CAD build for the part. Positions are in the model's coordinates, mm. A direction names the side the tool comes from. Round coordinates to 2 decimals unless told otherwise and drop trailing zeros. Order: outer loops, then holes, each group sorted by start corner. A loop starts at its lowest first (then second) coordinate and runs counter-clockwise, first axis right, second up. Notation, with made-up numbers: (88, 22) -> (135, 22) arc R14 ccw to (135, 48) -> close; hole circle Ø1 at (4, 28.5). An arc over 180 degrees is marked (long way). Return JSON: item names as keys, results as strings. Group by question number.
Q1. Flat gauge pins, fed straight in: pin 1 (1 mm diameter, centred on x = 54, z = 1.5, fed in from +Y); pin 2 (1 mm diameter, centred on y = 3.5, z = 1, fed in from -X); pin 3 (1.8 mm diameter, centred on y = 4.5, z = 2.5, fed in from +X); pin 4 (3 mm diameter, centred on x = 9.5, z = 2.5, fed in from +Y). Where does each tip first touch, or does it go through?
Q2. Cut at D-D (x = 5). Write the cut outline in (y, z), then the cut area to 3 significant figures.
Q3. Cut at C-C (x = 70). Write the cut outline in (y, z), then the cut area to 3 significant figures.
Q4. Cut at B-B (y = 33). Write the cut outline in (x, z).
Q5. Cut at A-A (z = 2). Write the cut outline in (x, y).
Q6. Probe line 1 along X through (y, z) = (4.5, 0.75); line 2 along Y through (x, z) = (70, -1); line 3 along Y through (x, z) = (5, -0.85). List the from-to ranges inside material, lowest first.
Q7. Which spindle directions (+Z, -Z, +X, -X, +Y, -Y) get a long thin tool onto all of the face, cutting with end or side? Do faces 1 (the flat face through (44.5, 12, 2)), 2 (the cylindrical face through (56.669, 19.474, 6.458)), 3 (the flat face through (55, 23, 2)). Say none if no direction does.
Q8. Mould opens along Y. For faces 4 (the flat face through (53.6, 18.7, 3.5)), 5 (the cylindrical face through (56.617, 5.67, 6.458)), 6 (the flat face through (47, 13, 9.5)), 7 (the flat face through (47, 15.5, 2)) say: +Y half, -Y half, draft (parallel to the pull), parting line (faces both ways), or undercut.
Autodesk Inventor part; units mm, degrees
ref_plane "YZ Plane" through (0, 0, 0) normal (1, 0, 0) x (0, 1, 0)
ref_plane "XZ Plane" through (0, 0, 0) normal (0, 1, 0) x (-1, 0, 0)
ref_plane "XY Plane" through (0, 0, 0) normal (0, 0, 1) x (1, 0, 0)
sketch "Skizze1" plane through (0, 0, 0) normal (0, 0, 1) x (1, 0, 0)
  line L0 (0, 0) -> (90, 0)
  line L1 (90, 0) -> (90, 37)
  line L2 (90, 37) -> (0, 37)
  line L3 (0, 37) -> (0, 0)
  dimension "d0" = 90
  dimension "d1" = 37
extrude "Extrusion1" add sketch "Skizze1" against normal blind 1.6
sketch "Skizze2" plane through (0, 0, 0) normal (0, 0, 1) x (1, 0, 0)
  circle A0 centre (5, 33) radius 1.75
  circle A1 centre (37.5, 5) radius 1.75
  circle A2 centre (70, 5) radius 1.75
  circle A3 centre (70, 23) radius 1.75
  line L0 (0, 0) -> (90, 0)
  line L1 (0, 37) -> (0, 0)
  line L2 (90, 0) -> (90, 37)
  dimension "d4" = 3.5
  dimension "d5" = 3.5
  dimension "d6" = 3.5
  dimension "d7" = 3.5
  dimension "d8" = 33
  dimension "d9" = 5
  dimension "d10" = 37.5
  dimension "d11" = 5
  dimension "d12" = 5
  dimension "d14" = 70
  dimension "d15" = 70
  dimension "d16" = 23
extrude "Extrusion2" cut sketch "Skizze2" against normal blind 1.6
sketch "Skizze3" plane through (0, 0, 0) normal (0, 0, 1) x (1, 0, 0)
  circle A0 centre (11.152, 35.373) radius 0.5
  line L0 (0, 0) -> (90, 0)
  line L1 (0, 37) -> (0, 0)
  circle A1 centre (12.889, 27.192) radius 0.5
  dimension "d19" = 1
  dimension "d20" = 35.373
  dimension "d21" = 11.152
  dimension "d22" = 1
  dimension "d23" = 27.192
  dimension "d24" = 12.889
extrude "Extrusion3" cut sketch "Skizze3" against normal blind 1.6
pattern_linear "Rechteckige Anordnung1" count 12 spacing 2.54 along (1, 0, 0) of "Extrusion3"
sketch "Skizze4" plane through (0, 0, 0) normal (0, 0, 1) x (1, 0, 0)
  line L0 (21.549, 28.192) -> (42.329, 28.192)
  line L1 (42.329, 28.192) -> (42.329, 26.192)
  line L2 (42.329, 26.192) -> (21.549, 26.192)
  line L3 (21.549, 26.192) -> (21.549, 28.192)
  circle A0 centre (23.049, 27.192) radius 0.5
  circle A1 centre (40.829, 27.192) radius 0.5
  point P0 (0, 0)
  dimension "d30" = 1
  dimension "d31" = 1
  dimension "d32" = 1
  dimension "d33" = 1
extrude "Extrusion4" add sketch "Skizze4" against normal blind 1.6 contours L0 L1 L2 L3 | A0 | A1
sketch "Skizze5" plane through (0, 0, 0) normal (0, 0, 1) x (1, 0, 0)
  line L0 (0, 37) -> (0, 0)
  line L1 (44.5, 15.5) -> (50.5, 15.5)
  line L2 (50.5, 15.5) -> (50.5, 9.5)
  line L3 (50.5, 9.5) -> (44.5, 9.5)
  line L4 (44.5, 9.5) -> (44.5, 15.5)
  line L5 (0, 0) -> (90, 0)
  line L6 (52, 23) -> (58, 23)
  line L7 (58, 23) -> (58, 17)
  line L8 (58, 17) -> (52, 17)
  line L9 (52, 17) -> (52, 23)
  line L10 (52, 8) -> (58, 8)
  line L11 (58, 8) -> (58, 2)
  line L12 (58, 2) -> (52, 2)
  line L13 (52, 2) -> (52, 8)
  line L14 (59.5, 15.5) -> (65.5, 15.5)
  line L15 (65.5, 15.5) -> (65.5, 9.5)
  line L16 (65.5, 9.5) -> (59.5, 9.5)
  line L17 (59.5, 9.5) -> (59.5, 15.5)
  line L18 (77, 23) -> (83, 23)
  line L19 (83, 23) -> (83, 17)
  line L20 (83, 17) -> (77, 17)
  line L21 (77, 17) -> (77, 23)
  line L22 (77, 8) -> (83, 8)
  line L23 (83, 8) -> (83, 2)
  line L24 (83, 2) -> (77, 2)
  line L25 (77, 2) -> (77, 8)
  point P0 (44.5, 12.5)
  point P1 (47.5, 9.5)
  point P2 (55, 17)
  point P3 (52, 20)
  point P4 (52, 5)
  point P5 (55, 2)
  point P6 (62.5, 9.5)
  point P7 (59.5, 12.5)
  point P8 (83, 20)
  point P9 (80, 17)
  point P10 (83, 5)
  point P11 (80, 2)
  dimension "d53" = 6
  dimension "d54" = 6
  dimension "d55" = 12.5
  dimension "d56" = 47.5
  dimension "d57" = 6
  dimension "d58" = 6
  dimension "d59" = 55
  dimension "d60" = 20
  dimension "d61" = 6
  dimension "d62" = 6
  dimension "d63" = 5
  dimension "d64" = 55
  dimension "d65" = 6
  dimension "d66" = 6
  dimension "d67" = 62.5
  dimension "d68" = 12.5
  dimension "d69" = 6
  dimension "d70" = 6
  dimension "d71" = 20
  dimension "d72" = 80
  dimension "d73" = 6
  dimension "d74" = 6
  dimension "d75" = 5
  dimension "d76" = 80
extrude "Extrusion5" add sketch "Skizze5" along normal blind 3.5
sketch "Skizze6" plane through (0, 0, 3.5) normal (0, 0, 1) x (1, 0, 0)
  line L0 (52, 17) -> (58, 17)
  line L1 (58, 17) -> (58, 23)
  line L2 (58, 23) -> (52, 23)
  line L3 (52, 23) -> (52, 17)
  line L4 (44.5, 9.5) -> (50.5, 9.5)
  line L5 (50.5, 9.5) -> (50.5, 15.5)
  line L6 (50.5, 15.5) -> (44.5, 15.5)
  line L7 (44.5, 15.5) -> (44.5, 9.5)
  line L8 (52, 2) -> (58, 2)
  line L9 (58, 2) -> (58, 8)
  line L10 (58, 8) -> (52, 8)
  line L11 (52, 8) -> (52, 2)
  line L12 (59.5, 9.5) -> (65.5, 9.5)
  line L13 (65.5, 9.5) -> (65.5, 15.5)
  line L14 (65.5, 15.5) -> (59.5, 15.5)
  line L15 (59.5, 15.5) -> (59.5, 9.5)
  line L16 (77, 17) -> (83, 17)
  line L17 (83, 17) -> (83, 23)
  line L18 (83, 23) -> (77, 23)
  line L19 (77, 23) -> (77, 17)
  line L20 (77, 2) -> (83, 2)
  line L21 (83, 2) -> (83, 8)
  line L22 (83, 8) -> (77, 8)
  line L23 (77, 8) -> (77, 2)
  circle A0 centre (47.5, 12.5) radius 1.75
  circle A1 centre (55, 20) radius 1.75
  circle A2 centre (62.5, 12.5) radius 1.75
  circle A3 centre (55, 5) radius 1.75
  circle A4 centre (80, 5) radius 1.75
  circle A5 centre (80, 20) radius 1.75
  point P0 (0, 0)
  dimension "d79" = 3.5
  dimension "d80" = 3.5
  dimension "d81" = 3.5
  dimension "d82" = 3.5
  dimension "d83" = 3.5
  dimension "d84" = 3.5
extrude "Buttons" add sketch "Skizze6" along normal blind 6 contours A0 | A1 | A2 | A3 | A4 | A5
sketch "Skizze7" plane through (0, 0, 0) normal (0, 0, 1) x (1, 0, 0)
  point P0 (0, 0)
properties part number "110_PICO_Daughterboard"
Solution:
{
 "1": {"pin 1": "stops at y = 23", "pin 2": "stops at x = 52", "pin 3": "stops at x = 83", "pin 4": "passes through"},
 "2": {"outline": "(0, -1.6) -> (31.25, -1.6) -> (31.25, 0) -> (0, 0) -> close; (34.75, -1.6) -> (37, -1.6) -> (37, 0) -> (34.75, 0) -> close", "area": "53.6 mm²"},
 "3": {"outline": "(0, -1.6) -> (3.25, -1.6) -> (3.25, 0) -> (0, 0) -> close; (6.75, -1.6) -> (21.25, -1.6) -> (21.25, 0) -> (6.75, 0) -> close; (24.75, -1.6) -> (37, -1.6) -> (37, 0) -> (24.75, 0) -> close", "area": "48.0 mm²"},
 "4": {"outline": "(0, -1.6) -> (3.25, -1.6) -> (3.25, 0) -> (0, 0) -> close; (6.75, -1.6) -> (90, -1.6) -> (90, 0) -> (6.75, 0) -> close"},
 "5": {"outline": "(44.5, 9.5) -> (50.5, 9.5) -> (50.5, 15.5) -> (44.5, 15.5) -> close; (52, 2) -> (58, 2) -> (58, 8) -> (52, 8) -> close; (52, 17) -> (58, 17) -> (58, 23) -> (52, 23) -> close; (59.5, 9.5) -> (65.5, 9.5) -> (65.5, 15.5) -> (59.5, 15.5) -> close; (77, 2) -> (83, 2) -> (83, 8) -> (77, 8) -> close; (77, 17) -> (83, 17) -> (83, 23) -> (77, 23) -> close"},
 "6": {"line 1": "x = 52 to 58, 77 to 83", "line 2": "y = 0 to 3.25, 6.75 to 21.25, 24.75 to 37", "line 3": "y = 0 to 31.25, 34.75 to 37"},
 "7": {"face 1": "+Z, -X, +Y, -Y", "face 2": "+Z", "face 3": "+Z, +X, -X, +Y"},
 "8": {"face 4": "undercut", "face 5": "undercut", "face 6": "draft", "face 7": "+Y half"}
}
